Work out the finished part from the listing and answer in its coordinate system (mm). Coordinates: 2 decimals unless noted, no trailing zeros. Order: outer loops, then holes, each group sorted by start corner. A loop starts at its lowest first (then second) coordinate and runs counter-clockwise, first axis right, second up. Notation, with made-up numbers: (21.5, -32) - (50.5, -32) arc R26 cw to (50.5, -1) - close; hole circle Ø4 at (50.5, 60.25). An arc over 180 degrees is marked (long way). Answer as a JSON object with one key per item and string values. Group by question number.
1) Section A-A (y = 2) is taken. Count the separate pieces of the cut face and the enclosed holes in it, plus the area to 3 significant figures.
2) Each of these flat-tipped pins is pushed along its axis until it touches: P1, Ø3, axis at x = 54.5, y = 4, coming from the +Z side; P2, Ø3.5, axis at x = 45.085, z = 42.545, coming from the -Y side; P3, Ø3, axis at x = -45, y = 4.5, coming from the +Z side; P4, Ø3, axis at y = 2.5, z = -62, coming from the +X side. Where does it stop, or does it pass through?
3) Section B-B (x = -43.5) is taken. Give the vertices of the cut face in (y, z), plus the area to 3 significant figures.
4) Find the intervals of material crossed by line 1 along X through (y, z) = (5, 42.5); line 2 along Z through (x, y) = (51, 6.25); line 3 along Z through (x, y) = (-26, 4), in increasing order.
5) Section C-C (z = 49.5) is taken. Give the vertices of the cut face in (x, y).
from build123d import *

# Parameters (mm, degrees)
SKETCH1_W           = 114.3
SKETCH1_H           = 127
BOSS_EXTRUDE1_DEPTH = 6.35
CAVITY2_START       = 50.8
CAVITY2_OUTLINE_W   = 6.35
CAVITY2_OUTLINE_H   = 29.633333333
CAVITY2_OUTLINE_H_2 = 7.281333333
CAVITY2_OUTLINE_H_3 = 30.734
CAVITY2_DEPTH       = 6.35
CAVITY2_START_2     = -57.15
CAVITY2_2_OUTLINE_W = 6.35
CAVITY2_2_OUTLINE_H = 6.35
CAVITY2_2_DEPTH     = 22.86
CAVITY2_START_3     = -11.43
CAVITY2_3_OUTLINE_W = 6.35
CAVITY2_3_OUTLINE_H = 6.35
CAVITY2_3_DEPTH     = 22.86
CAVITY2_START_4     = 34.29
CAVITY2_4_OUTLINE_W = 6.35
CAVITY2_4_OUTLINE_H = 6.35
CAVITY2_4_DEPTH     = 16.51
SKETCH2_R           = 1.905
CUT_EXTRUDE1_DEPTH  = 86.666183527


# Read off the part's stored shape, not the designer's step: Cavity2
with BuildPart() as part:
    # Sketch1 → Boss-Extrude1 (new body)
    with BuildSketch(Plane(origin=(0, 0, 0), x_dir=(1, 0, 0), z_dir=(0, 1, 0))):
        Rectangle(SKETCH1_W, SKETCH1_H)
    extrude(amount=BOSS_EXTRUDE1_DEPTH)

    # Cavity2 outline → Cavity2 (cut)
    with BuildSketch(Plane.YZ.offset(CAVITY2_START)):
        with Locations((3.175, 48.683333334)):
            Rectangle(CAVITY2_OUTLINE_W, CAVITY2_OUTLINE_H)
        with Locations((3.175, 0.592666666)):
            Rectangle(CAVITY2_OUTLINE_W, CAVITY2_OUTLINE_H_2)
        with Locations((3.175, -48.133)):
            Rectangle(CAVITY2_OUTLINE_W, CAVITY2_OUTLINE_H_3)
    extrude(amount=CAVITY2_DEPTH, mode=Mode.SUBTRACT)

    # Cavity2 2 outline → Cavity2 2 (cut)
    with BuildSketch(Plane.YZ.offset(CAVITY2_START_2)):
        with Locations((3.175, 60.325)):
            Rectangle(CAVITY2_2_OUTLINE_W, CAVITY2_2_OUTLINE_H)
        with Locations((3.175, -60.325)):
            Rectangle(CAVITY2_2_OUTLINE_W, CAVITY2_2_OUTLINE_H)
    extrude(amount=CAVITY2_2_DEPTH, mode=Mode.SUBTRACT)

    # Cavity2 3 outline → Cavity2 3 (cut)
    with BuildSketch(Plane.YZ.offset(CAVITY2_START_3)):
        with Locations((3.175, 60.325)):
            Rectangle(CAVITY2_3_OUTLINE_W, CAVITY2_3_OUTLINE_H)
        with Locations((3.175, -60.325)):
            Rectangle(CAVITY2_3_OUTLINE_W, CAVITY2_3_OUTLINE_H)
    extrude(amount=CAVITY2_3_DEPTH, mode=Mode.SUBTRACT)

    # Cavity2 4 outline → Cavity2 4 (cut)
    with BuildSketch(Plane.YZ.offset(CAVITY2_START_4)):
        with Locations((3.175, 60.325)):
            Rectangle(CAVITY2_4_OUTLINE_W, CAVITY2_4_OUTLINE_H)
        with Locations((3.175, -60.325)):
            Rectangle(CAVITY2_4_OUTLINE_W, CAVITY2_4_OUTLINE_H)
    extrude(amount=CAVITY2_4_DEPTH, mode=Mode.SUBTRACT)

    # Sketch2 → Cut-Extrude1 (cut, through all)
    with BuildSketch(Plane.XZ):
        with Locations(Location((45.085, -42.545, 0), (0, 0, 270))):
            Circle(SKETCH2_R)
        with Locations(Location((-24.765, -42.545, 0), (0, 0, 270))):
            Circle(SKETCH2_R)
        with Locations(Location((45.085, 42.545, 0), (0, 0, 270))):
            Circle(SKETCH2_R)
        with Locations(Location((-24.765, 42.545, 0), (0, 0, 270))):
            Circle(SKETCH2_R)
    extrude(amount=-CUT_EXTRUDE1_DEPTH, mode=Mode.SUBTRACT)


solid = part.part
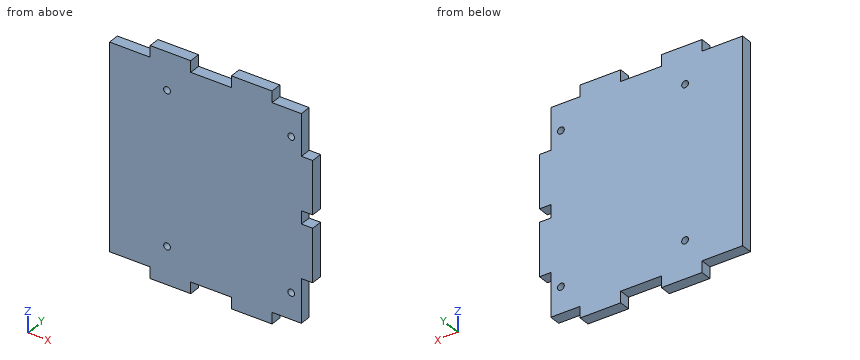
Report:
{
 "1": {"separate pieces": "1", "enclosed holes": "4", "area": "13,300 mm²"},
 "2": {"P1": "stops at z = 33.87", "P2": "passes through", "P3": "stops at z = 57.15", "P4": "stops at x = 34.29"},
 "3": {"outline": "(0, -57.15) - (6.35, -57.15) - (6.35, 57.15) - (0, 57.15) - close", "area": "726 mm²"},
 "4": {"line 1": "x = -57.15 to -26.67, -22.86 to 43.18, 46.99 to 50.8", "line 2": "z = -32.77 to -3.05, 4.23 to 33.87", "line 3": "z = -63.5 to -44, -41.09 to 41.09, 44 to 63.5"},
 "5": {"outline": "(-57.15, 0) - (50.8, 0) - (50.8, 6.35) - (-57.15, 6.35) - close"}
}
